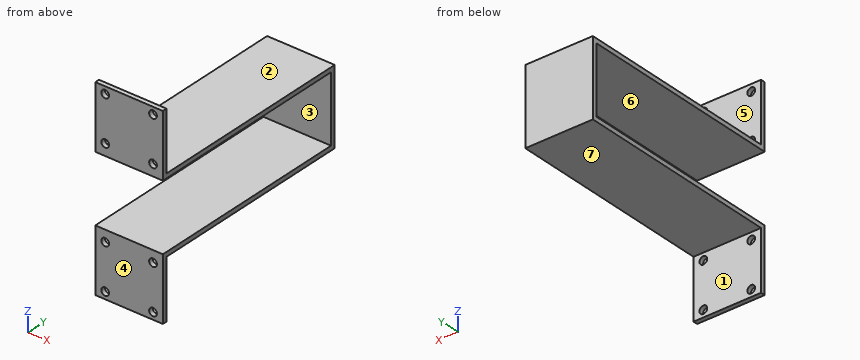
Autodesk Inventor part; units mm, degrees
ref_plane "YZ Plane" through (0, 0, 0) normal (1, 0, 0) x (0, 1, 0)
ref_plane "XZ Plane" through (0, 0, 0) normal (0, 1, 0) x (-1, 0, 0)
ref_plane "XY Plane" through (0, 0, 0) normal (0, 0, 1) x (1, 0, 0)
sketch "Sketch1" plane through (0, 0, 0) normal (1, 0, 0) x (0, 1, 0)
  line L0 (0, 69) -> (0, 23.825)
  line L1 (0, 23.825) -> (146.825, 23.825)
  line L2 (146.825, 23.825) -> (146.825, -23.825)
  line L3 (146.825, -23.825) -> (0, -23.825)
  line L4 (0, -23.825) -> (0, -69)
  line L5 (0, -69) -> (3.175, -69)
  line L6 (3.175, -69) -> (3.175, -27)
  line L7 (3.175, -27) -> (150, -27)
  line L8 (150, -27) -> (150, 27)
  line L9 (150, 27) -> (3.175, 27)
  line L10 (3.175, 27) -> (3.175, 69)
  line L11 (3.175, 69) -> (0, 69)
  line L12 (6.6614, 27) -> (6.6614, 23.825) construction
  line L13 (146.825, 0) -> (150, 0) construction
  line L14 (6.6614, -23.825) -> (6.6614, -27) construction
  line L15 (-30, 0) -> (180, 0) construction
  line L16 (106.5396, 5.913) -> (72.5659, 5.913) construction
  line L17 (114.8237, 26.913) -> (65.8343, 26.913) construction
  point P0 (0, 0)
  dimension "d0" = 3.175
  dimension "d3" = 150
  dimension "d4" = 29.738
  dimension "d5" = 21
  dimension "d24" = 42
  dimension "d25" = 54
extrude "Extrusion1" add sketch "Sketch1" along normal mid plane 48
sketch "Sketch2" plane through (-24, 0, 23.825) normal (0, -1, 0) x (1, 0, 0)
  line L0 (0, 0) -> (0, 45.175)
  line L1 (0, 0) -> (48, 0)
  line L2 (48, 45.175) -> (48, 0)
  line L3 (48, 45.175) -> (0, 45.175)
  line L4 (0, -92.825) -> (0, -47.65)
  line L5 (0, -92.825) -> (48, -92.825)
  line L6 (48, -47.65) -> (48, -92.825)
  line L7 (0, -47.65) -> (48, -47.65)
  line L8 (0, 0) -> (48, 0)
  line L9 (0, 0) -> (0, 45.175)
  line L10 (24, 72.775) -> (24, -120.425)
  point P0 (24, -23.825)
  point P1 (41, 40.175)
  dimension "d9" = 5
  dimension "d10" = 17
hole "Hole1" at (17, 0, 64) direction (0, 1, 0) diameter 5.5 end through all
pattern_linear "Rectangular Pattern1" count 2 spacing 32 along (0, 0, -1) count 2 spacing 34 along (-1, 0, 0) of "Hole1"
mirror "Mirror1" about plane through (0, 0, 0) normal (0, 0, 1) of "Hole1", "Rectangular Pattern1"
equation "\"d25\" = Gap"
properties part number "Sheet Metal Arm v2"
Verification items for the finished model (mm, model axes). Face numbers are marked on the shaded views. A direction names the side the tool comes from. Round coordinates to 2 decimals unless told otherwise and drop trailing zeros. Loops run counter-clockwise (first coordinate to the right, second up) from the corner with the lowest first, then second, coordinate; pieces in that order, holes last. Notation, with made-up numbers: (-33.75, 65.5) - (19.25, 65.5) arc R22 cw to (19.25, 83.5) - close; hole circle Ø11 at (33, 61). An arc over 180 degrees is marked (long way). Use one line per item in the form item = value.
1. Section check D-D on x = -0.5. Record the cut outline in (y, z) (3 decimals), and give its area (3 significant figures).
A:
outline = (0, -69) - (3.175, -69) - (3.175, -27) - (150, -27) - (150, 27) - (3.175, 27) - (3.175, 69) - (0, 69) - (0, 23.825) - (146.825, 23.825) - (146.825, -23.825) - (0, -23.825) - close
area = 1,370 mm²
2. Gauge pin test, flat ends, axial feed: pin 1 Ø24 at (x, z) = (-6.5, -8.5) entering from -Y (3 decimals); pin 2 Ø24 at (x, y) = (-8, 55) entering from -Z; pin 3 Ø6.5 at (x, z) = (17, -64) entering from +Y (3 decimals); pin 4 Ø1 at (x, z) = (12, -31.5) entering from -Y. Record the tip position at first contact, or that the pin passes through.
A:
pin_1 = 146.825
pin_2 = -27
pin_3 = 3.175
pin_4 = 0
3. Access from +Z, -Z, +X, -X, +Y, -Y to the whole of each face (thin tool, end or side, straight path). Record for the marked faces 4, 5, 6 and 7.
A:
face_4 = +Z, -Z, +X, -X, -Y
face_5 = +Z, +X, -X, +Y
face_6 = +X, -X, -Y
face_7 = -Z, +X, -X, +Y
4. Scan lines: probe 1 along Z at (x, y) = (17, 0.75) (3 decimals); probe 2 along X at (y, z) = (1.95, 64); probe 3 along Z at (x, y) = (-13, 50.5) (3 decimals). Record each from-to range of solid material in increasing order.
A:
probe_1 = -69 to -66.75, -61.25 to -34.75, -29.25 to -23.825, 23.825 to 29.25, 34.75 to 61.25, 66.75 to 69
probe_2 = -24 to -19.75, -14.25 to 14.25, 19.75 to 24
probe_3 = -27 to -23.825, 23.825 to 27
5. Section check A-A on x = 17. Record the cut outline in (y, z) (3 decimals).
A:
outline = (0, -69) - (3.175, -69) - (3.175, -66.75) - (0, -66.75) - close; (0, -61.25) - (3.175, -61.25) - (3.175, -34.75) - (0, -34.75) - close; (0, -29.25) - (3.175, -29.25) - (3.175, -27) - (150, -27) - (150, 27) - (3.175, 27) - (3.175, 29.25) - (0, 29.25) - (0, 23.825) - (146.825, 23.825) - (146.825, -23.825) - (0, -23.825) - close; (0, 34.75) - (3.175, 34.75) - (3.175, 61.25) - (0, 61.25) - close; (0, 66.75) - (3.175, 66.75) - (3.175, 69) - (0, 69) - close
6. Draft check along Z on the marked faces 1, 2 and 3. Enter one of: pulls with the +Z half, pulls with the -Z half, needs draft (parallel to the pull), parting line crosses it, or undercut.
A:
face_1 = needs draft
face_2 = pulls with the +Z half
face_3 = undercut
7. Section check C-C on y = 16. Record the cut outline in (x, z) (3 decimals).
A:
outline = (-24, -27) - (24, -27) - (24, -23.825) - (-24, -23.825) - close; (-24, 23.825) - (24, 23.825) - (24, 27) - (-24, 27) - close
8. Section check B-B on z = -64. Record the cut outline in (x, y) (3 decimals).
A:
outline = (-24, 0) - (-19.75, 0) - (-19.75, 3.175) - (-24, 3.175) - close; (-14.25, 0) - (14.25, 0) - (14.25, 3.175) - (-14.25, 3.175) - close; (19.75, 0) - (24, 0) - (24, 3.175) - (19.75, 3.175) - close
